Source: CAD feature listing. Evaluate the final solid. Frame: model axes, mm. Face numbers are marked on the shaded views. A direction names the side the tool comes from. Give positions to 0.01 mm unless a question says otherwise; leave off trailing zeros. Order: outer loops, then holes, each group sorted by start corner. A loop starts at its lowest first (then second) coordinate and runs counter-clockwise, first axis right, second up.
```python
from build123d import *

# Parameters (mm, degrees)
BOSS_EXTRU_1_DEPTH      = 10
BOSS_EXTRU_2_DEPTH      = 10
BOSS_EXTRU_2_DEPTH_BACK = 20
ESQUISSE2_W             = 69
ESQUISSE2_H             = 10
ESQUISSE4_W             = 19
ESQUISSE4_H             = 23.50582434
ESQUISSE4_R             = 4.1
BOSS_EXTRU_3_DEPTH      = 10
ESQUISSE5_W             = 5
ESQUISSE5_H             = 30
BOSS_EXTRU_4_DEPTH      = 5
ESQUISSE6_W             = 69
ESQUISSE6_H             = 5
BOSS_EXTRU_5_DEPTH      = 15
ESQUISSE7_R             = 5.448918283
BOSS_EXTRU_6_DEPTH      = 5
CHANFREIN2_SIZE         = 5
ESQUISSE8_R             = 2.1
ENL_V_MAT_EXTRU_1_DEPTH = 5
ESQUISSE9_R             = 1.6
ENL_V_MAT_EXTRU_2_DEPTH = 68
ESQUISSE10_W            = 50
ESQUISSE10_H            = 5
BOSS_EXTRU_7_DEPTH      = 15
CHANFREIN3_SIZE         = 5
ESQUISSE11_R            = 2.1
ENL_V_MAT_EXTRU_3_DEPTH = 10
CONG_1_R                = 2
CONG_2_R                = 5


with BuildPart() as part:
    # Esquisse1 → Boss.-Extru.1 (new body)
    with BuildSketch(Plane.XY):
        Polygon((0, 0), (0, 81), (-69, 81), (-69, 66), (-64, 66), (-64, 71), (-50, 71), (-50, 0), align=None)
    extrude(amount=BOSS_EXTRU_1_DEPTH)

    # Esquisse2 → Boss.-Extru.2 (add, two sides: drawn at the far end of the back side and taken through both)
    with BuildSketch(Plane.XY.offset(10).offset(-BOSS_EXTRU_2_DEPTH_BACK)):
        with Locations((-34.5, 76)):
            Rectangle(ESQUISSE2_W, ESQUISSE2_H)
    extrude(amount=BOSS_EXTRU_2_DEPTH + BOSS_EXTRU_2_DEPTH_BACK)

    # Esquisse4 → Boss.-Extru.3 (add)
    with BuildSketch(Plane.XY.offset(10)):
        with Locations((-59.5, 11.75291217)):
            Rectangle(ESQUISSE4_W, ESQUISSE4_H)
        with Locations((-57, 12)):
            Circle(ESQUISSE4_R, mode=Mode.SUBTRACT)
    extrude(amount=-BOSS_EXTRU_3_DEPTH)

    # Esquisse5 → Boss.-Extru.4 (add)
    with BuildSketch(Plane.XZ.offset(-71)):
        with Locations((-66.5, 5)):
            Rectangle(ESQUISSE5_W, ESQUISSE5_H)
    extrude(amount=BOSS_EXTRU_4_DEPTH)

    # Esquisse6 → Boss.-Extru.5 (add)
    with BuildSketch(Plane.XY.offset(10)):
        with Locations((-34.5, 2.5)):
            Rectangle(ESQUISSE6_W, ESQUISSE6_H)
    extrude(amount=BOSS_EXTRU_5_DEPTH)

    # Esquisse7 → Boss.-Extru.6 (add)
    with BuildSketch(Plane.XY.offset(10)):
        with Locations((-57, 12)):
            Circle(ESQUISSE7_R)
    extrude(amount=-BOSS_EXTRU_6_DEPTH)

    # Chanfrein2
    chanfrein2_edges = [part.edges().sort_by_distance(p)[0] for p in [
        (-34.5, 5, 10),
    ]]
    chamfer(chanfrein2_edges, length=CHANFREIN2_SIZE)

    # Esquisse8 → Enlèv. mat.-Extru.1 (cut)
    with BuildSketch(Plane(origin=(0, 5, 0), x_dir=(1, 0, 0), z_dir=(0, 1, 0))):
        with Locations(Location((-15, -20, 0), (0, 0, 180))):
            Circle(ESQUISSE8_R)
        with Locations(Location((-54, -20, 0), (0, 0, 180))):
            Circle(ESQUISSE8_R)
    extrude(amount=-ENL_V_MAT_EXTRU_1_DEPTH, mode=Mode.SUBTRACT)

    # Esquisse9 → Enlèv. mat.-Extru.2 (cut)
    with BuildSketch(Plane.ZY.offset(50)):
        with Locations(Location((5, 63.50582434, 0), (0, 0, 270))):
            Circle(ESQUISSE9_R)
        with Locations(Location((5, 43.50582434, 0), (0, 0, 270))):
            Circle(ESQUISSE9_R)
    extrude(amount=-ENL_V_MAT_EXTRU_2_DEPTH, mode=Mode.SUBTRACT)

    # Esquisse10 → Boss.-Extru.7 (add)
    with BuildSketch(Plane(origin=(0, 0, 0), x_dir=(-1, 0, 0), z_dir=(0, 0, -1))):
        with Locations((25, 13.5)):
            Rectangle(ESQUISSE10_W, ESQUISSE10_H)
    extrude(amount=BOSS_EXTRU_7_DEPTH)

    # Chanfrein3
    chanfrein3_edges = [part.edges().sort_by_distance(p)[0] for p in [
        (-25, 11, 0),
    ]]
    chamfer(chanfrein3_edges, length=CHANFREIN3_SIZE)

    # Esquisse11 → Enlèv. mat.-Extru.3 (cut)
    with BuildSketch(Plane(origin=(0, 16, 0), x_dir=(1, 0, 0), z_dir=(0, 1, 0))):
        with Locations(Location((-10, 10, 0), (0, 0, 270))):
            Circle(ESQUISSE11_R)
        with Locations(Location((-40, 10, 0), (0, 0, 270))):
            Circle(ESQUISSE11_R)
    extrude(amount=-ENL_V_MAT_EXTRU_3_DEPTH, mode=Mode.SUBTRACT)

    # Congé1
    cong_1_edges = [part.edges().sort_by_distance(p)[0] for p in [
        (-10, 16, -12.1),
        (-40, 16, -12.1),
    ]]
    fillet(cong_1_edges, radius=CONG_1_R)

    # Congé2
    cong_2_edges = [part.edges().sort_by_distance(p)[0] for p in [
        (-34.5, 10, 10),
        (-34.5, 5, 15),
        (-32, 71, -10),
        (0, 71, -5),
        (0, 71, 15),
        (-32, 71, 20),
        (-34.5, 81, 20),
        (-34.5, 81, -10),
        (0, 81, 5),
        (-69, 81, 5),
        (-69, 66, 5),
    ]]
    fillet(cong_2_edges, radius=CONG_2_R - 0.0001)  # a hair under: the kernel refuses the full size


solid = part.part
```
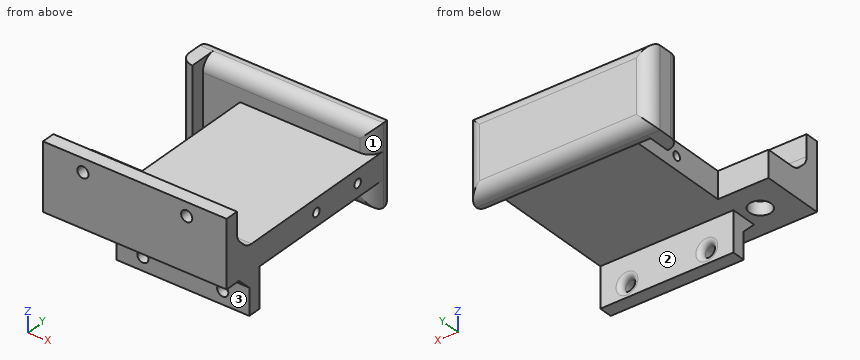
1) Material intervals for L1, parallel to Z at x = -15, y = 1.2; L2, parallel to Y at x = -54, z = 9; L3, parallel to Z at x = -16.5, y = 29, sorted ascending.
Report:
L1: z = 0 to 17.9, 22.1 to 25
L2: y = 0 to 23.51, 71 to 81
L3: z = 0 to 10
2) Reachability of the marked faces 1, 2 and 3 from +Z, -Z, +X, -X, +Y, -Y: full face, straight path, thin tool, end or side. Return the list, or none.
Report:
face 1: +Z, +X
face 2: -Z, +X, -X
face 3: -Z, +X, -X, -Y
3) Section query A-A, the plane x = -10. Count the separate pieces of the cut face and the enclosed holes in it, and give its area (3 significant figures).
Report:
separate pieces: 2
enclosed holes: 2
area: 1,130 mm2
4) Pin query (flat end, axial travel): pin 1 (12 mm diameter, centred on x = -44.5, y = 50.5, fed in from -Z); pin 2 (5 mm diameter, centred on x = -40, z = -10, fed in from -Y); pin 3 (8.5 mm diameter, centred on x = -51, z = 19.5, fed in from +Y); pin 4 (2.5 mm diameter, centred on y = 63.51, z = 5, fed in from +X). Return the tip coordinate at first contact, or that it passes through.
Report:
pin 1: stops at z = 0
pin 2: stops at y = 11
pin 3: stops at y = 80.99
pin 4: passes through
5) Section query C-C, the plane z = 21. Return the cut outline in (x, y).
Report:
outline: (-69, 0) - (-55.85, 0) - (-55.85, 5) - (-69, 5) - close; (-52.15, 0) - (-16.85, 0) - (-16.85, 5) - (-52.15, 5) - close; (-13.15, 0) - (0, 0) - (0, 5) - (-13.15, 5) - close
